Input: part model. Units: mm. Frame: model coordinates. A direction names the side the tool comes from. Round coordinates to 2 decimals unless told otherwise and drop trailing zeros. Loops run counter-clockwise (first coordinate to the right, second up) from the corner with the lowest first, then second, coordinate; pieces in that order, holes last.
1) First-contact query: pin 1 (3 mm diameter, centred on x = 15.5, y = -14.5, fed in from -Z); pin 2 (3 mm diameter, centred on y = 3, z = -3, fed in from -X); pin 3 (1.5 mm diameter, centred on x = 13.5, y = 9.5, fed in from -Z). Flat tips, straight axial feed; report the tip coordinate or a pass-through.
2) Access query for faces 1 (the face through (-1.5, 11.4, -0.1)), 2 (the face through (-10, 14, 0)), 3 (the face through (0, -21, 2)). Directions: +Z, -Z, +X, -X, +Y, -Y. A direction counts if a zero-diameter tool reaches every point of the face in a straight line with its end or side. Return the directions, or none.
3) Section C-C, the plane z = 3. Return loops of the section in (x, y), and give its area (3 significant figures).
4) Draft query along X for faces 4 (the face through (-21, 0, 2)), 5 (the face through (-14.985, 0.66, -3.972)), 6 (the face through (12.526, -12.648, 1.972)). Return one class per face: pulls with the +X half, pulls with the -X half, needs draft (parallel to the pull), parting line crosses it, or undercut.
5) Ray query, line 1 along Y through (x, z) = (14, 2.85); line 2 along Z through (x, y) = (11.5, -15); line 3 along X through (y, z) = (6, 2.5). Return the intervals inside material, ascending.
6) Section D-D, the plane z = -3.5. Return loops of the section in (x, y).
7) Section A-A, the plane x = 0. Return loops of the section in (y, z).
from build123d import *

# Parameters (mm, degrees)
SKETCH1_W           = 42
SKETCH1_H           = 42
SKETCH1_R           = 2
SKETCH1_R_2         = 11.5
BOSS_EXTRUDE1_DEPTH = 4
SKETCH2_R           = 15
SKETCH2_R_2         = 11.5
BOSS_EXTRUDE2_DEPTH = 6
SKETCH3_R           = 11.5
SKETCH3_R_2         = 9.5
BOSS_EXTRUDE3_DEPTH = 2
FILLET1_R           = 2


with BuildPart() as part:
    # Sketch1 → Boss-Extrude1 (new body)
    with BuildSketch(Plane.XY):
        Rectangle(SKETCH1_W, SKETCH1_H)
        with Locations((-14, -14)):
            Circle(SKETCH1_R, mode=Mode.SUBTRACT)
        with Locations((14, 14)):
            Circle(SKETCH1_R, mode=Mode.SUBTRACT)
        with Locations((14, -14)):
            Circle(SKETCH1_R, mode=Mode.SUBTRACT)
        with Locations((-14, 14)):
            Circle(SKETCH1_R, mode=Mode.SUBTRACT)
        Circle(SKETCH1_R_2, mode=Mode.SUBTRACT)
    extrude(amount=BOSS_EXTRUDE1_DEPTH)

    # Sketch2 → Boss-Extrude2 (add)
    with BuildSketch(Plane.XY):
        Circle(SKETCH2_R)
        Circle(SKETCH2_R_2, mode=Mode.SUBTRACT)
    extrude(amount=-BOSS_EXTRUDE2_DEPTH)

    # Sketch3 → Boss-Extrude3 (add)
    with BuildSketch(Plane(origin=(0, 0, -6), x_dir=(-1, 0, 0), z_dir=(0, 0, -1))):
        Circle(SKETCH3_R)
        Circle(SKETCH3_R_2, mode=Mode.SUBTRACT)
    extrude(amount=-BOSS_EXTRUDE3_DEPTH)

    # Fillet1
    fillet1_edges = [part.edges().sort_by_distance(p)[0] for p in [
        (-15, 0, 0),
    ]]
    fillet(fillet1_edges, radius=FILLET1_R)


solid = part.part
Final values:
1. pin 1: stops at z = 0
1. pin 2: stops at x = -14.92
1. pin 3: stops at z = -0.43
2. face 1: +Z
2. face 2: -Z
2. face 3: +Z, -Z, +X, -X, -Y
3. outline: (-21, -21) - (21, -21) - (21, 21) - (-21, 21) - close; hole circle Ø4 at (-14, -14); hole circle Ø4 at (-14, 14); hole circle Ø23 at (0, 0); hole circle Ø4 at (14, -14); hole circle Ø4 at (14, 14)
3. area: 1,300 mm2
4. face 4: pulls with the -X half
4. face 5: parting line crosses it
4. face 6: undercut
5. line 1: y = -21 to -16, -12 to 12, 16 to 21
5. line 2: z = 0 to 4
5. line 3: x = -21 to -9.81, 9.81 to 21
6. outline: circle Ø30 at (0, 0); hole circle Ø23 at (0, 0)
7. outline: (-21, 0) - (-17, 0) arc R2 cw to (-15, -2) - (-15, -6) - (-9.5, -6) - (-9.5, -4) - (-11.5, -4) - (-11.5, 4) - (-21, 4) - close; (9.5, -6) - (15, -6) - (15, -2) arc R2 cw to (17, 0) - (21, 0) - (21, 4) - (11.5, 4) - (11.5, -4) - (9.5, -4) - close
